Geometry check sheet. Reference: the model listing, model coordinates, mm. A direction names the side the tool comes from. Round coordinates to 2 decimals unless told otherwise and drop trailing zeros. Write each loop counter-clockwise with the first axis right and the second up, starting at its lowest first coordinate (ties: lowest second). Pieces come first, ordered by that corner, then holes. Notation, with made-up numbers: (76, 0.25) - (128, 0.25) arc R13 ccw to (128, 25.25) - close; hole circle Ø9 at (56, 4.5). An arc over 180 degrees is marked (long way). Return JSON: item names as keys, results as strings. Group by question number.
Solid Edge part; units mm, degrees
sketch "Sketch1" plane through (0, 0, 0) normal (0, 0, 1) x (1, 0, 0)
  line L0 (25, -40) -> (-25, -40)
  line L1 (-25, -40) -> (-25, 40)
  line L2 (-25, 40) -> (25, 40)
  line L3 (25, 40) -> (25, -40)
  dimension "D1" = 25
extrude "Protrusion1" add sketch "Sketch1" along normal blind 5.5
hole "Hole_1" at (5, -0.0052, 5.5) direction (0, 0, -1) diameter 12 depth 140
hole "Hole_2" at (-2.75, 13.4182, 5.5) direction (0, 0, -1) diameter 3.2 end through all
pattern_circular "Pattern1" count 6 over 360 about axis through (5.0085, -0.0003, 5.5) along (0, 0, -1) of "Hole_2"
hole "Hole_8" at (-20, -35, 5.5) direction (0, 0, -1) diameter 3.2 end through all
hole "Hole6" at (-20, 35, 5.5) direction (0, 0, -1) diameter 3.2 end through all
hole "Hole7" at (20, 35, 5.5) direction (0, 0, -1) diameter 3.2 end through all
hole "Hole8" at (20, -35, 5.5) direction (0, 0, -1) diameter 3.2 end through all
fillet "Round_1" radius 2 4 edges at (25, 40, 2.75) (-25, 40, 2.75) (-25, -40, 2.75) (25, -40, 2.75)
sketch "Sketch2" plane through (0, 0, 5.5) normal (0, 0, 1) x (-1, 0, 0)
  line L0 (25, -10) -> (45, -10)
  line L1 (45, -10) -> (45, 10)
  line L2 (45, 10) -> (25, 10)
  line L3 (25, 10) -> (25, -10)
  dimension "D1" = 45
  dimension "D2" = 45
extrude "ExtrudedProtrusion_2" add sketch "Sketch2" against normal blind 5
hole "Hole_12" at (-30, -0.0101, 5.5) direction (0, 0, -1) diameter 9 end up to next
hole "Hole_13" at (-39, -0.0101, 5.5) direction (0, 0, -1) diameter 3.2 end up to next
hole "Hole9" at (-21, -0.0101, 5.5) direction (0, 0, -1) diameter 3.2 end up to next
fillet "Round_2" radius 2 4 edges at (-25, -10, 3) (-45, -10, 3) (-45, 10, 3) (-25, 10, 3)
properties material "木材, アッシュ"
1. Material ranges on line 1 along X through (y, z) = (35, 1.9); line 2 along Y through (x, z) = (-2.75, 2.9); line 3 along Y through (x, z) = (-21, 1.25), recorded low to high.
2. Section check A-A (x = -39). Enter the section's corners in (y, z).
3. Tool access check on faces 1 (the face through (-3.72, 14.69, 2.79)), 2 (the face through (-35, -10, 3)). Record the directions out of +Z, -Z, +X, -X, +Y, -Y that give a thin tool (end or side, any length) a straight path to the whole face; none if there is none.
4. Section check D-D (x = 5). Enter the section's corners in (y, z), and give its area (3 significant figures).
5. Depth check by flat-ended pin: pin 1 Ø5 at (x, y) = (-39, -0.01) entering from -Z; pin 2 Ø2.5 at (x, z) = (-33.5, 3) entering from +Y. Enter the tip coordinate at first touch or a pass-through.
6. Section check C-C (z = 4.1). State how many separate pieces and enclosed holes the cut face has, and give its area (3 significant figures).
7. Mould release check, pull along Y, two halves, no side actions. Record for faces 3 (the face through (-44.43, 9.4, 2.96)), 4 (the face through (21.08, -33.82, 2.79)), 5 (the face through (-5, 1, 0)): pulls with the +Y half, pulls with the -Y half, needs draft (parallel to the pull), parting line crosses it, or undercut.
8. Section check B-B (y = -35). Enter the section's corners in (x, z), and give its area (3 significant figures).
Result sheet:
{
 "1": {"line 1": "x = -25 to -21.6, -18.4 to 18.4, 21.6 to 25", "line 2": "y = -40 to -15.03, -11.83 to 11.82, 15.02 to 40", "line 3": "y = -40 to -36.25, -33.75 to -1.61, 1.59 to 33.75, 36.25 to 40"},
 "2": {"outline": "(-10, 0.5) - (-1.61, 0.5) - (-1.61, 5.5) - (-10, 5.5) - close; (1.59, 0.5) - (10, 0.5) - (10, 5.5) - (1.59, 5.5) - close"},
 "3": {"face 1": "+Z, -Z", "face 2": "+Z, -Z, -X, -Y"},
 "4": {"outline": "(-40, 0) - (-6.01, 0) - (-6.01, 5.5) - (-40, 5.5) - close; (5.99, 0) - (40, 0) - (40, 5.5) - (5.99, 5.5) - close", "area": "374 mm²"},
 "5": {"pin 1": "stops at z = 0.5", "pin 2": "stops at y = 10"},
 "6": {"separate pieces": "1", "enclosed holes": "14", "area": "4,120 mm²"},
 "7": {"face 3": "pulls with the +Y half", "face 4": "undercut", "face 5": "needs draft"},
 "8": {"outline": "(-25, 0) - (-21.6, 0) - (-21.6, 5.5) - (-25, 5.5) - close; (-18.4, 0) - (18.4, 0) - (18.4, 5.5) - (-18.4, 5.5) - close; (21.6, 0) - (25, 0) - (25, 5.5) - (21.6, 5.5) - close", "area": "240 mm²"}
}
